Part model, mm, in its own coordinate system. A direction names the side the tool comes from. Round coordinates to 2 decimals unless told otherwise and drop trailing zeros. Write each loop counter-clockwise with the first axis right and the second up, starting at its lowest first coordinate (ties: lowest second). Pieces come first, ordered by that corner, then holes. Notation, with made-up numbers: (66.5, -29) -> (76.5, -29) arc R24 cw to (76.5, -19) -> close; hole circle Ø2 at (-19, 53). An arc over 180 degrees is marked (long way). Return JSON: item names as keys, results as strings. Group by question number.
Autodesk Inventor part; units mm, degrees
ref_plane "YZ Plane" through (0, 0, 0) normal (1, 0, 0) x (0, 1, 0)
ref_plane "XZ Plane" through (0, 0, 0) normal (0, 1, 0) x (-1, 0, 0)
ref_plane "XY Plane" through (0, 0, 0) normal (0, 0, 1) x (1, 0, 0)
sketch "Эскиз1" plane through (0, 0, 0) normal (0, 1, 0) x (-1, 0, 0)
  line L0 (9, 8.8) -> (9, -8.8) construction
  line L1 (-9, -8.8) -> (-9, 8.8) construction
  line L2 (-9, 8.8) -> (9, -8.8) construction
  line L3 (9, 8.8) -> (-9, -8.8) construction
  line L4 (9, 0) -> (9, 0.5)
  line L5 (9, 0.5) -> (-9, 0.5)
  line L6 (9, 0) -> (9, -0.4719)
  line L7 (9, -0.4719) -> (-9, -0.4719)
  line L8 (-9, 0.5) -> (-9, -0.4719)
  line L9 (9, 0) -> (9, 4.3404) construction
  line L10 (9, 0) -> (9, -4.4046) construction
  line L11 (9, 4.3404) -> (-9, 4.3404)
  line L12 (-9, 4.3404) -> (-9, 8.8)
  line L13 (-9, 8.8) -> (9, 8.8)
  line L14 (9, 8.8) -> (9, 4.3404)
  line L15 (9, -4.4046) -> (-9, -4.4046)
  line L16 (-9, -4.4046) -> (-9, -8.8)
  line L17 (-9, -8.8) -> (9, -8.8)
  line L18 (9, -8.8) -> (9, -4.4046)
  point P0 (0, 0)
  dimension "d0" = 18
  dimension "d1" = 17.6
  dimension "d2" = 0.5
extrude "Выдавливание1" add sketch "Эскиз1" along normal blind 18.4
sketch "Эскиз4" plane through (9, 0, 8.8) normal (1, 0, 0) x (0, 0, -1)
  line L0 (13.2046, 0) -> (17.6, 0)
  line L1 (14.5773, 0) -> (21.0298, 0)
  line L2 (21.0298, 0) -> (21.0298, 4.45)
  line L3 (21.0298, 4.45) -> (14.5773, 4.45)
  line L4 (14.5773, 4.45) -> (14.5773, 0)
  line L5 (14.5773, 18.4) -> (21.6, 18.4)
  line L6 (21.6, 18.4) -> (21.6, 13.95)
  line L7 (21.6, 13.95) -> (14.5773, 13.95)
  line L8 (14.5773, 13.95) -> (14.5773, 18.4)
  line L9 (4.4596, 18.4) -> (0, 18.4)
  line L10 (2.5726, 18.4) -> (-5.1704, 18.4)
  line L11 (-5.1704, 18.4) -> (-5.1704, 13.95)
  line L12 (-5.1704, 13.95) -> (2.5726, 13.95)
  line L13 (2.5726, 13.95) -> (2.5726, 18.4)
  line L14 (4.4596, 0) -> (0, 0)
  line L15 (2.5726, 0) -> (-6.491, 0)
  line L16 (-6.491, 0) -> (-6.491, 4.45)
  line L17 (-6.491, 4.45) -> (2.5726, 4.45)
  line L18 (2.5726, 4.45) -> (2.5726, 0)
  line L19 (20.6227, 11.95) -> (14.5773, 11.95)
  line L20 (14.5773, 11.95) -> (14.5773, 6.45)
  line L21 (14.5773, 6.45) -> (20.6227, 6.45)
  line L22 (20.6227, 6.45) -> (20.6227, 11.95)
  line L23 (17.6, 0) -> (17.6, 18.4)
  line L24 (20.6227, 11.95) -> (14.5773, 6.45) construction
  line L25 (14.5773, 11.95) -> (20.6227, 6.45) construction
  line L26 (-2.5726, 11.95) -> (2.5726, 11.95)
  line L27 (2.5726, 11.95) -> (2.5726, 6.45)
  line L28 (2.5726, 6.45) -> (-2.5726, 6.45)
  line L29 (-2.5726, 6.45) -> (-2.5726, 11.95)
  line L30 (0, 0) -> (0, 18.4)
  line L31 (-2.5726, 11.95) -> (2.5726, 6.45) construction
  line L32 (2.5726, 11.95) -> (-2.5726, 6.45) construction
  point P0 (8.8, 0)
  point P1 (17.6, 9.2)
  point P2 (0, 9.2)
  dimension "d12" = 5.5
  dimension "d41" = 2
  dimension "d42" = 2
  dimension "d43" = 2
extrude "Выдавливание2" cut sketch "Эскиз4" against normal blind 12.4
sketch "Эскиз6" plane through (9, 0, 4.3404) normal (0, 0, -1) x (-1, 0, 0)
  line L0 (9, 0) -> (9, 18.4) construction
  line L1 (18, 18.4) -> (0, 18.4)
  line L2 (9, 9.2) -> (7.5, 9.2) construction
  circle A0 centre (7.5, 9.2) radius 5.5
  dimension "d16" = 1.5
  dimension "d53" = 11
sketch "Эскиз7" plane through (-9, 0, -8.8) normal (0, 0, -1) x (-1, 0, 0)
  line L0 (-18, 13.95) -> (-5.6, 13.95)
  line L1 (-18, 0) -> (-18, 18.4) construction
  line L2 (-21, -3) -> (-15, -3) construction
  line L3 (-15, -3) -> (-15, 3) construction
  line L4 (-15, 3) -> (-21, 3) construction
  line L5 (-21, 3) -> (-21, -3) construction
  line L6 (-21, -3) -> (-15, 3) construction
  line L7 (-15, -3) -> (-21, 3) construction
  line L8 (-21.3737, 21.4) -> (-15.3737, 21.4) construction
  line L9 (-15.3737, 21.4) -> (-15.3737, 15.4) construction
  line L10 (-15.3737, 15.4) -> (-21.3737, 15.4) construction
  line L11 (-21.3737, 15.4) -> (-21.3737, 21.4) construction
  line L12 (-21.3737, 21.4) -> (-15.3737, 15.4) construction
  line L13 (-15.3737, 21.4) -> (-21.3737, 15.4) construction
  arc A0 (-18, 3) -> (-15, 0) centre (-15, 3) ccw
  arc A1 (-15.3737, 18.4) -> (-18, 13.95) centre (-15.3737, 15.4) ccw
  line L14 (-18, 3) -> (-18, 0)
  line L15 (-15, 0) -> (-18, 0)
  line L16 (-15.3737, 18.4) -> (-18, 18.4)
  line L17 (-18, 13.95) -> (-18, 18.4)
  point P0 (-9, 0)
  dimension "d21" = 6
  dimension "d22" = 6
extrude "Выдавливание3" add sketch "Эскиз6" along normal up to surface (8.745 mm away)
extrude "Выдавливание4" cut sketch "Эскиз7" against normal blind 23
ref_plane "РабПлоскость1" through (-3.4, 9.2, 8.8) normal (0, -1, 0) x (0, 0, -1)
sketch "Эскиз9" plane through (-3.4, 9.2, 8.8) normal (0, -1, 0) x (0, 0, -1)
  line L0 (-0.964, 17.4) -> (18.536, 17.4)
  line L1 (18.536, 17.4) -> (18.536, 0.5)
  line L2 (18.536, 0.5) -> (-0.964, 0.5)
  line L3 (-0.964, 0.5) -> (-0.964, 17.4)
  line L4 (2.3726, 13.4) -> (14.7773, 13.4)
  line L5 (14.7773, 13.4) -> (14.7773, 4.5)
  line L6 (14.7773, 4.5) -> (2.3726, 4.5)
  line L7 (2.3726, 4.5) -> (2.3726, 13.4)
  line L8 (8.786, 13.2041) -> (8.786, 18.9436) construction
  line L9 (0, 0) -> (0, 12.4)
  line L10 (17.6, -5.6) -> (13.2046, -5.6)
  point P0 (8.8, 3.4)
  point P1 (17.6, 0)
  point P2 (2.5726, 12.4)
  point P3 (14.5773, 12.4)
  dimension "d30" = 8.786
  dimension "d31" = 9.75
  dimension "d32" = 9.75
  dimension "d33" = 23
  dimension "d34" = 0.5
  dimension "d35" = 0.2
  dimension "d36" = 0.2
  dimension "d37" = 4
  dimension "d38" = 4
extrude "Выдавливание5" add sketch "Эскиз9" along normal mid plane 5
sketch "Эскиз10" plane through (-9, 0, 4.3404) normal (-1, 0, 0) x (0, 0, 1)
  line L0 (4.4596, 6.45) -> (4.4596, 11.95)
  line L1 (4.4596, 9.2) -> (-13.9375, 9.2) construction
  line L2 (-14.0763, 6.7) -> (-14.0763, 11.7)
  line L3 (1, 9.2) -> (2.9596, 9.2) construction
  line L4 (1, 8.2) -> (2.9596, 8.2)
  line L5 (2.9596, 10.2) -> (1, 10.2)
  arc A0 (1, 10.2) -> (1, 8.2) centre (1, 9.2) ccw
  arc A1 (2.9596, 8.2) -> (2.9596, 10.2) centre (2.9596, 9.2) ccw
  line L6 (0, 0) -> (0, 18.4)
  line L7 (4.4596, 0) -> (4.4596, 18.4)
  line L8 (-9.745, 9.2) -> (-11.6404, 9.2) construction
  line L9 (-9.745, 10.2) -> (-11.6404, 10.2)
  line L10 (-11.6404, 8.2) -> (-9.745, 8.2)
  arc A2 (-9.745, 8.2) -> (-9.745, 10.2) centre (-9.745, 9.2) ccw
  arc A3 (-11.6404, 10.2) -> (-11.6404, 8.2) centre (-11.6404, 9.2) ccw
  line L11 (-8.745, 0) -> (-8.745, 18.4)
  line L12 (-13.1404, 0) -> (-13.1404, 18.4)
  line L13 (-4.8123, 0) -> (-4.8123, 18.4)
  line L14 (-3.8404, 0) -> (-3.8404, 3)
  line L15 (-4.8123, 0) -> (-3.8404, 0)
  line L16 (-3.8404, 0) -> (-3.8404, 3)
  line L17 (-3.8404, 3) -> (-4.8123, 3)
  line L18 (-4.8123, 3) -> (-4.8123, 0)
  line L19 (-4.8123, 3) -> (-4.8123, 16.85)
  line L20 (-3.8404, 18.4) -> (-4.8123, 18.4)
  line L21 (-4.8123, 18.4) -> (-4.8123, 15.4)
  line L22 (-4.8123, 15.4) -> (-3.8404, 15.4)
  line L23 (-3.8404, 15.4) -> (-3.8404, 18.4)
  line L24 (8.1135, -3.7823) -> (-17.89, -3.7823)
  line L25 (-17.89, -3.7823) -> (-17.89, 22.1054)
  line L26 (-17.89, 22.1054) -> (8.1135, 22.1054)
  line L27 (8.1135, 22.1054) -> (8.1135, -3.7823)
  point P0 (-4.3404, 0)
  point P1 (1.9798, 9.2)
  point P2 (-10.6927, 9.2)
  point P3 (-4.8123, 3)
  dimension "d44" = 2
  dimension "d45" = 1
  dimension "d46" = 1.5
  dimension "d47" = 1
  dimension "d48" = 1.5
  dimension "d49" = 3
  dimension "d50" = 3
extrude "Выдавливание6" cut sketch "Эскиз10" against normal blind 3
sketch "Эскиз11" plane through (-6, 0, 4.3404) normal (-1, 0, 0) x (0, 0, 1)
  line L0 (-4.3263, -2.8057) -> (-4.3263, 20.2349) construction
  line L1 (5.7896, 9.2) -> (-19.3839, 9.2) construction
  line L2 (2.1737, 14.2) -> (-10.8263, 14.2) construction
  line L3 (-10.8263, 14.2) -> (-10.8263, 4.2) construction
  line L4 (-10.8263, 4.2) -> (2.1737, 4.2) construction
  line L5 (2.1737, 4.2) -> (2.1737, 14.2) construction
  line L6 (2.1737, 14.2) -> (-10.8263, 4.2) construction
  line L7 (-10.8263, 14.2) -> (2.1737, 4.2) construction
  circle A0 centre (2.1737, 4.2) radius 0.35
  circle A1 centre (-10.8263, 4.2) radius 0.35
  circle A2 centre (-10.8263, 14.2) radius 0.35
  circle A3 centre (2.1737, 14.2) radius 0.35
  point P0 (-4.3404, 0)
  point P1 (-4.3263, 9.2)
  dimension "d54" = 13
  dimension "d55" = 10
  dimension "d56" = 0.7
  dimension "d57" = 0.7
  dimension "d58" = 0.7
  dimension "d59" = 0.7
extrude "Выдавливание7" add sketch "Эскиз11" along normal blind 7.5
properties part number "UU10.5"
Item 1: Cut at A-A (z = 5). Write the cut outline in (x, y).
Item 2: Flat gauge pins, fed straight in: P1, Ø6, axis at x = -7, y = 8.5, coming from the +Z side; P2, Ø3, axis at x = 2.5, z = 8, coming from the +Y side; P3, Ø6, axis at x = -5, y = 5.5, coming from the -Z side; P4, Ø4, axis at y = 16.5, z = -2.5, coming from the +X side. Where does each tip first touch, or does it go through?
Item 3: Cut at B-B (x = 1.5). State how many separate pieces and enclosed holes the cut face has, then the cut area to 3 significant figures.
Item 4: Cut at C-C (y = 13). Write the cut outline in (x, z).
Item 5: Two-plate mould, pull along Z, no slides. Class faces 5 (the face through (-4, 7, 4.34)), 6 (the face through (-8, 10.2, 6)), 7 (the face through (3, 16, -5.777)): released by +Z, released by -Z, zero draft, split by the parting line, or undercut.
Item 6: Which spindle directions (+Z, -Z, +X, -X, +Y, -Y) get a long thin tool onto all of the face, cutting with end or side? Do faces 1 (the face through (-3.4, 16, -7)), 2 (the face through (-9, 9, 6)), 3 (the face through (-3.4, 9, -7)), 4 (the face through (-3.4, 2, 8)). Say none if no direction does.
Item 7: Wall check: L1, parallel to Z at x = -2.5, y = 3.25; L2, parallel to Y at x = 8.25, z = -7.25; L3, parallel to X at y = 7.5, z = -5. Give the ranges that are in metal, low to high.
Checks:
{
 "1": {"outline": "(-9, 8.26) -> (-6, 8.26) -> (-6, 0) -> (6, 0) arc R3 ccw to (9, 3) -> (9, 16.85) arc R3 ccw to (6.37, 18.4) -> (-6, 18.4) -> (-6, 10.14) -> (-9, 10.14) -> close; (10, 6.7) -> (14, 6.7) -> (14, 11.7) -> (10, 11.7) -> close"},
 "2": {"P1": "stops at z = 8.8", "P2": "stops at y = 13.95", "P3": "stops at z = -9.74", "P4": "stops at x = 9"},
 "3": {"separate pieces": "3", "enclosed holes": "0", "area": "221 mm2"},
 "4": {"outline": "(-6, -8.8) -> (9, -8.8) -> (9, -4.4) -> (5.48, -4.4) -> (5.48, -0.47) -> (9, -0.47) -> (9, 0.5) -> (5.48, 0.5) -> (5.48, 4.34) -> (9, 4.34) -> (9, 8.8) -> (-6, 8.8) -> (-6, 4.34) -> (-2.48, 4.34) -> (-2.48, 0.5) -> (-6, 0.5) -> (-6, -0.47) -> (-2.48, -0.47) -> (-2.48, -4.4) -> (-6, -4.4) -> close"},
 "5": {"face 5": "undercut", "face 6": "zero draft", "face 7": "released by -Z"},
 "6": {"face 1": "-Z, +X, +Y", "face 2": "+Z, -Z, -X", "face 3": "-Z", "face 4": "+Z, +X, -Y"},
 "7": {"L1": "z = -5.78 to -4.4, -0.47 to 0.5, 4.34 to 6.23", "L2": "y = 4.45 to 6.45, 6.7 to 11.7, 11.95 to 13.95", "L3": "x = -6 to 9, 10 to 14"}
}
